For this review, take the finished solid that the model builds, in its own axes (mm). Round coordinates to 2 decimals unless told otherwise and drop trailing zeros. Write each loop counter-clockwise with the first axis right and the second up, starting at its lowest first coordinate (ties: lowest second). Pieces come first, ordered by that corner, then holes. Notation, with made-up numbers: M 37,-3 L 80,-3 A13 cw 80,10 Z; hole C 62,54.5 d8. An arc over 180 degrees is marked long. Answer in a Markdown table with one row per item.
```python
from build123d import *

# Parameters (mm, degrees)
F0_W     = 7
F0_H     = 13
F1_DEPTH = 40
F2_R     = 6
F5_D     = 2


with BuildPart() as f1:
    # F0 (on Top) → F1 (new body)
    with BuildSketch(Plane.XY):
        Rectangle(F0_W, F0_H)
    extrude(amount=F1_DEPTH)

    # F2
    f2_edges = [f1.edges().sort_by_distance(p)[0] for p in [
        (0, 6.5, 40),
        (0, -6.5, 40),
        (0, 6.5, 0),
        (0, -6.5, 0),
    ]]
    fillet(f2_edges, radius=F2_R)

    # F5 (through all)
    with Locations(Plane(origin=(-3.5, 0, 0), x_dir=(0, -1, 0), z_dir=(-1, 0, 0))):
        with Locations((0, 4), (0, 36)):
            Hole(F5_D / 2)


solid = f1.part
```
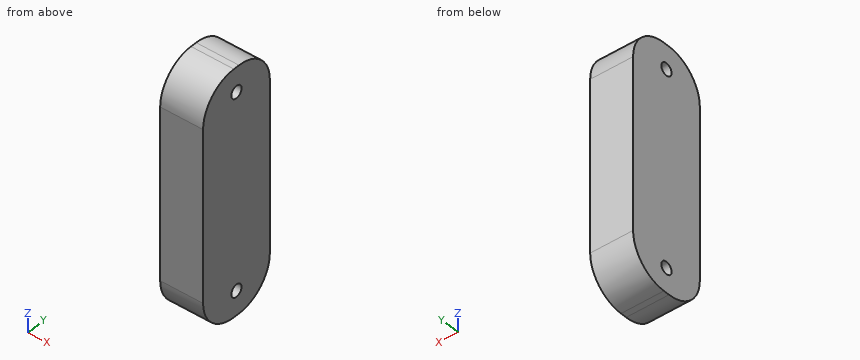
Q1. Take a section at A-A (y = 0). State the section outline as (x, z) points, then the cut area to 3 significant figures.
Found:
| item | result |
|---|---|
| outline | M -3.5,0 L 3.5,0 L 3.5,3 L -3.5,3 Z; M -3.5,5 L 3.5,5 L 3.5,35 L -3.5,35 Z; M -3.5,37 L 3.5,37 L 3.5,40 L -3.5,40 Z |
| area | 252 mm² |
Q2. Take a section at B-B (x = -1.25). State the section outline as (y, z) points, then the cut area to 3 significant figures.
Found:
| item | result |
|---|---|
| outline | M -6.5,6 A6 ccw -0.5,0 L 0.5,0 A6 ccw 6.5,6 L 6.5,34 A6 ccw 0.5,40 L -0.5,40 A6 ccw -6.5,34 Z; hole C 0,4 d2; hole C 0,36 d2 |
| area | 483 mm² |
Q3. For probe 1 along Z at (x, y) = (-1, 0); probe 2 along Z at (x, y) = (0.25, 0.75); probe 3 along Z at (x, y) = (-2.25, 4.25), list the stretches that pass through material, from the lowest coordinate up.
Found:
| item | result |
|---|---|
| probe 1 | 0 to 3, 5 to 35, 37 to 40 |
| probe 2 | 0.01 to 3.34, 4.66 to 35.34, 36.66 to 39.99 |
| probe 3 | 1.32 to 38.68 |
Q4. Insertion check: P1, Ø1, axis at x = 2.5, z = 4.5, coming from the -Y side; P2, Ø3, axis at x = 2, y = -2.5, coming from the -Z side. Each pin has a flat end and moves straight along its axis. Give the tip position at first contact, or say it passes through.
Found:
| item | result |
|---|---|
| P1 | y = -6.42 |
| P2 | z = 0.02 |
Q5. Take a section at C-C (z = 4). State the section outline as (x, y) points, then the cut area to 3 significant figures.
Found:
| item | result |
|---|---|
| outline | M -3.5,-6.16 L 3.5,-6.16 L 3.5,-1 L -3.5,-1 Z; M -3.5,1 L 3.5,1 L 3.5,6.16 L -3.5,6.16 Z |
| area | 72.2 mm² |
